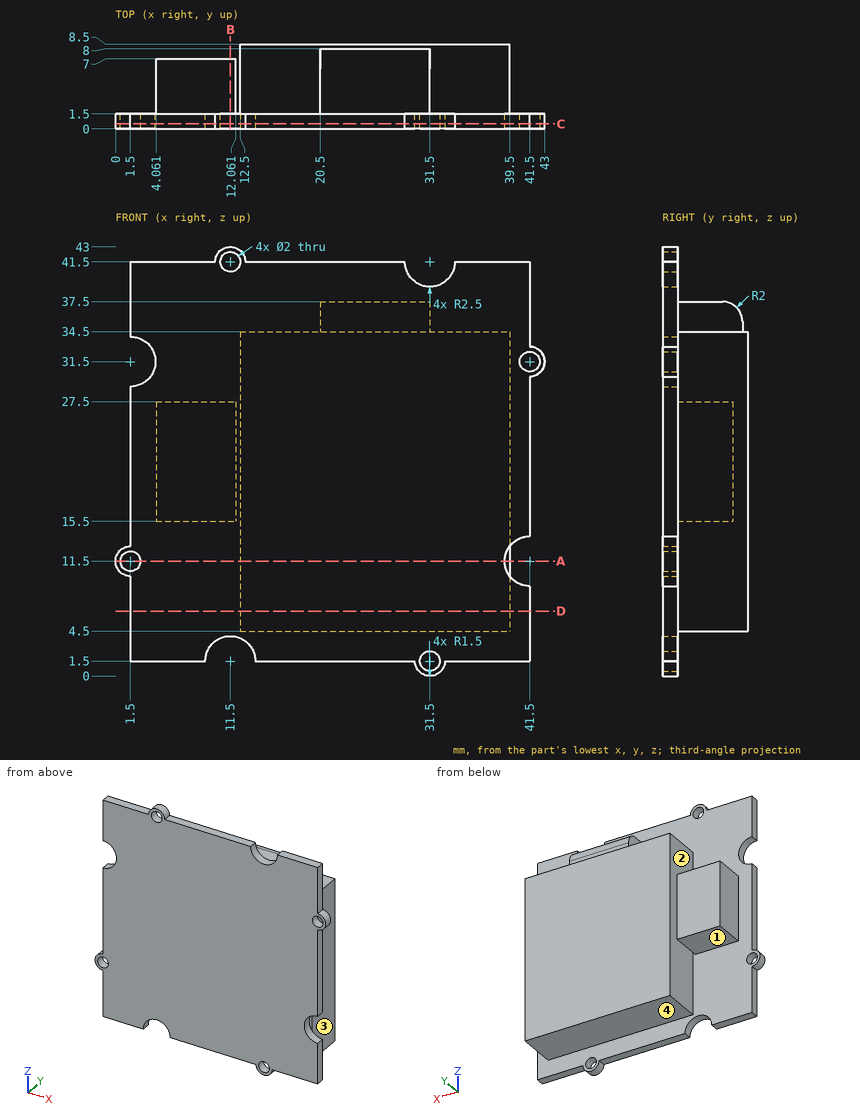
Design review of the part shown in the three views and the two pictorial views. Dimensions are in mm from the part's minimum x, y and z. A direction names the side the tool comes from. Give positions to 0.01 mm unless a question says otherwise; leave off trailing zeros. Write each loop counter-clockwise with the first axis right and the second up, starting at its lowest first coordinate (ties: lowest second). Pieces come first, ordered by that corner, then holes.
(1) Clearance check with flat-ended pins moving along their axes: pin 1 Ø4 at (x, z) = (14.5, 36) entering from +Y; pin 2 Ø1.3 at (x, y) = (27, 3.5) entering from +Z; pin 3 Ø4 at (y, z) = (7.5, 16.5) entering from +X; pin 4 Ø2 at (y, z) = (6, 30.5) entering from -X. State where each tip first meets the part, or that it passes through.
Checked values:
pin 1: stops at y = 8.5
pin 2: stops at z = 37.5
pin 3: stops at x = 39.5
pin 4: stops at x = 12.5
(2) Add section C-C (y = 0.5). Give the boundary of the cut face in (x, z).
Checked values:
outline: (1.5, 1.5) - (9, 1.5) arc R2.5 cw to (14, 1.5) - (30, 1.5) arc R1.5 ccw to (33, 1.5) - (41.5, 1.5) - (41.5, 9) arc R2.5 cw to (41.5, 14) - (41.5, 30) arc R1.5 ccw to (41.5, 33) - (41.5, 41.5) - (34, 41.5) arc R2.5 cw to (29, 41.5) - (13, 41.5) arc R1.5 ccw to (10, 41.5) - (1.5, 41.5) - (1.5, 34) arc R2.5 cw to (1.5, 29) - (1.5, 13) arc R1.5 ccw to (1.5, 10) - close; hole circle Ø2 at (1.5, 11.5); hole circle Ø2 at (11.5, 41.5); hole circle Ø2 at (31.5, 1.5); hole circle Ø2 at (41.5, 31.5)
(3) Add section A-A (z = 11.5). Give the boundary of the cut face in (x, y).
Checked values:
outline: (0, 0) - (0.5, 0) - (0.5, 1.5) - (0, 1.5) - close; (2.5, 0) - (39, 0) - (39, 1.5) - (39.5, 1.5) - (39.5, 8.5) - (12.5, 8.5) - (12.5, 1.5) - (2.5, 1.5) - close
(4) Add section B-B (x = 11.5). Give the boundary of the cut face in (y, z).
Checked values:
outline: (0, 4) - (1.5, 4) - (1.5, 15.5) - (7, 15.5) - (7, 27.5) - (1.5, 27.5) - (1.5, 40.5) - (0, 40.5) - close; (0, 42.5) - (1.5, 42.5) - (1.5, 43) - (0, 43) - close
(5) Wall thickness on line 1 along Z through (x, y) = (31.5, 0.45); line 2 along X through (y, z) = (1.25, 6); line 3 along Z through (x, y) = (11.5, 1.1): over which ranges is each line inside the solid? List them lowest first.
Checked values:
line 1: z = 0 to 0.5, 2.5 to 39
line 2: x = 1.5 to 41.5
line 3: z = 4 to 40.5, 42.5 to 43
(6) Tool access review of the marked faces 1, 2, 3 and 4: name each direction out of +Z, -Z, +X, -X, +Y, -Y from which nothing blocks a thin tool from reaching the whole face with its end or side.
Checked values:
face 1: -Z, -X, +Y
face 2: +Z, -Z, +Y
face 3: +Z, -Z, +X, +Y
face 4: -Z, +X, -X, +Y
(7) Add section D-D (z = 6.5). Give the boundary of the cut face in (x, y), and give its area (3 significant figures).
Checked values:
outline: (1.5, 0) - (41.5, 0) - (41.5, 1.5) - (39.5, 1.5) - (39.5, 8.5) - (12.5, 8.5) - (12.5, 1.5) - (1.5, 1.5) - close
area: 249 mm2
